The drawing under review shows one solid part. Ordinate dimensions are in mm from its lowest x, y, z. Round coordinates to 2 decimals unless told otherwise and drop trailing zeros. Order: outer loops, then holes, each group sorted by start corner. A loop starts at its lowest first (then second) coordinate and runs counter-clockwise, first axis right, second up. Notation, with made-up numbers: M -28.5,43 L -9.5,43 A31 cw -9.5,77 Z; hole C 58,16 d3. An arc over 180 degrees is marked long. Answer as a JSON object with one key per item and string values. Group by question number.
1. Add section A-A on y = 6. Give the number of separate pieces and of enclosed holes in the cut face, and give its area (3 significant figures).
2. Add section C-C on x = 92.17. State the section outline as (y, z) points.
3. Add section D-D on z = 19.74. State the section outline as (x, y) points.
4. To check wall thickness, follow probe 1 along X at (y, z) = (4.65, 4.5); probe 2 along X at (y, z) = (7.3, 52.76); probe 3 along X at (y, z) = (6.6, 47.68). State the ranges of each line that lie inside material, in increasing order. Write a range as [from, to].
5. Clearance check with flat-ended pins moving along their axes: P1, Ø2, axis at x = 12.5, z = 32.5, coming from the +Y side; P2, Ø3, axis at x = 92, z = 5, coming from the +Y side. State where each tip first meets the part, or that it passes through.
6. Add section B-B on z = 52.76. State the section outline as (x, y) points, and give its area (3 significant figures).
7. Mouldability with a two-part tool opening along X and no side actions: class the marked faces 1 and 2 as released by +X, released by -X, zero draft, split by the parting line, or undercut.
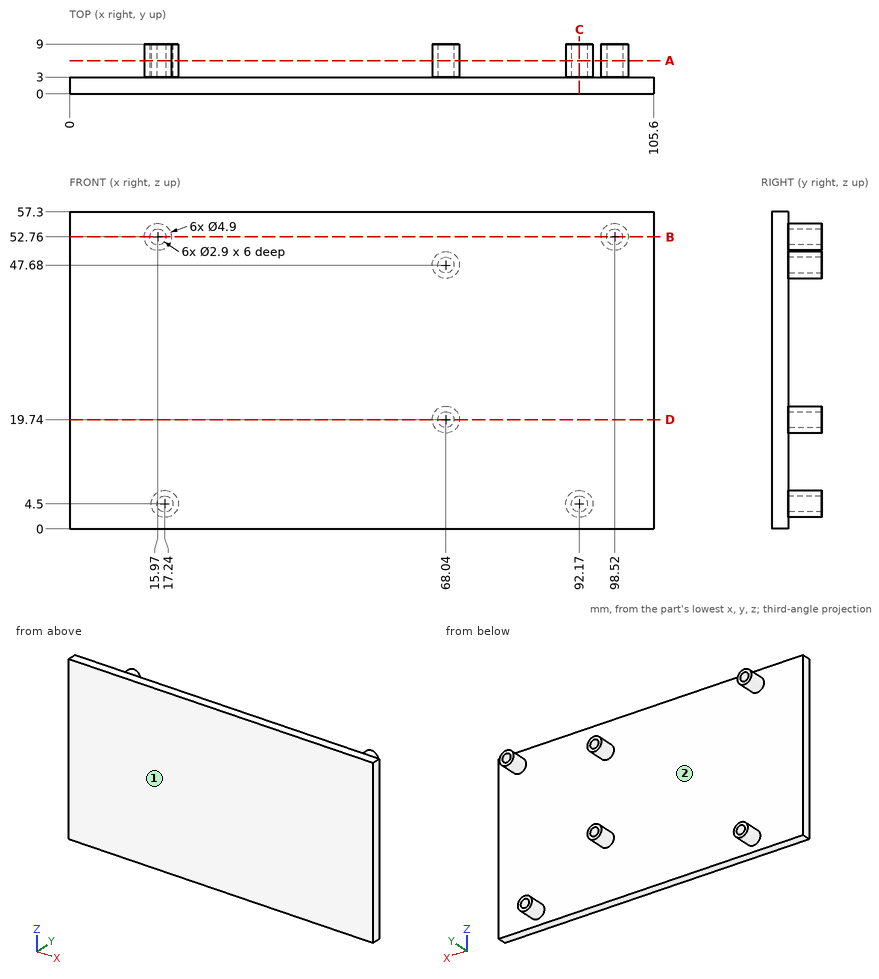
Recorded:
{
 "1": {"separate pieces": "6", "enclosed holes": "6", "area": "73.5 mm²"},
 "2": {"outline": "M 0,0 L 3,0 L 3,2.05 L 9,2.05 L 9,3.05 L 3,3.05 L 3,5.95 L 9,5.95 L 9,6.95 L 3,6.95 L 3,57.3 L 0,57.3 Z"},
 "3": {"outline": "M 0,0 L 105.6,0 L 105.6,3 L 70.49,3 L 70.49,9 L 69.49,9 L 69.49,3 L 66.59,3 L 66.59,9 L 65.59,9 L 65.59,3 L 0,3 Z"},
 "4": {"probe 1": "x = [14.79, 15.79], [18.69, 19.69], [89.72, 90.72], [93.62, 94.62]", "probe 2": "x = [13.52, 14.52], [17.42, 18.42], [96.07, 97.07], [99.97, 100.97]", "probe 3": "x = [65.59, 66.59], [69.49, 70.49]"},
 "5": {"P1": "stops at y = 3", "P2": "stops at y = 9"},
 "6": {"outline": "M 0,0 L 105.6,0 L 105.6,3 L 100.97,3 L 100.97,9 L 99.97,9 L 99.97,3 L 97.07,3 L 97.07,9 L 96.07,9 L 96.07,3 L 18.42,3 L 18.42,9 L 17.42,9 L 17.42,3 L 14.52,3 L 14.52,9 L 13.52,9 L 13.52,3 L 0,3 Z", "area": "341 mm²"},
 "7": {"face 1": "zero draft", "face 2": "undercut"}
}
